Work out the finished part from the listing and answer in its coordinate system (mm). A direction names the side the tool comes from. Give positions to 0.01 mm unless a question says otherwise; leave off trailing zeros. Order: outer loops, then holes, each group sorted by start corner. A loop starts at its lowest first (then second) coordinate and runs counter-clockwise, first axis right, second up. Notation, with made-up numbers: (-32, 60.5) -> (-22, 60.5) arc R19 ccw to (-22, 81.5) -> close; hole circle Ø6 at (-31.5, 6.5). An arc over 180 degrees is marked (long way). Use a Markdown table: item, result. Add a question column.
```python
from build123d import *

# Parameters (mm, degrees)
BOSS_EXTRUDE1_DEPTH = 3.175
SKETCH3_R           = 3.3782
CUT_EXTRUDE2_DEPTH  = 4.175
SKETCH4_R           = 3.3782
CUT_EXTRUDE3_DEPTH  = 4.175
CHAMFER1_SIZE       = 3.175
CUT_EXTRUDE4_DEPTH  = 4.175


with BuildPart() as part:
    # Sketch1 → Boss-Extrude1 (new body)
    with BuildSketch(Plane(origin=(0, 0, 0), x_dir=(0, 0, -1), z_dir=(1, 0, 0))):
        with BuildLine():
            Line((118.405818623, 279.4), (147.442069819, 279.4))
            ThreePointArc((147.442069819, 279.4), (151.349937349, 278.055104531), (153.602474695, 274.590101219))
            Line((153.602474695, 274.590101219), (215.9, 25.4))
            Line((215.9, 25.4), (215.9, 0))
            Line((215.9, 0), (0, 0))
            Line((0, 0), (0, 25.4))
            Line((0, 25.4), (112.615117065, 275.655815701))
            ThreePointArc((112.615117065, 275.655815701), (114.95795187, 278.382421106), (118.405818623, 279.4))
        make_face()
    extrude(amount=BOSS_EXTRUDE1_DEPTH)

    # Sketch3 → Cut-Extrude2 (cut, through all)
    with BuildSketch(Plane(origin=(3.175, 0, 0), x_dir=(0, 0, -1), z_dir=(1, 0, 0))):
        with Locations((146.05, 244.475)):
            Circle(SKETCH3_R)
        with Locations((129.249479175, 225.425)):
            Circle(SKETCH3_R)
        with Locations((129.249479175, 263.525)):
            Circle(SKETCH3_R)
    extrude(amount=-CUT_EXTRUDE2_DEPTH, mode=Mode.SUBTRACT)

    # Sketch4 → Cut-Extrude3 (cut, through all)
    with BuildSketch(Plane(origin=(3.175, 0, 0), x_dir=(0, 0, -1), z_dir=(1, 0, 0))):
        with Locations((12.7, 12.7)):
            Circle(SKETCH4_R)
        with Locations((107.95, 12.7)):
            Circle(SKETCH4_R)
        with Locations((203.2, 12.7)):
            Circle(SKETCH4_R)
    extrude(amount=-CUT_EXTRUDE3_DEPTH, mode=Mode.SUBTRACT)

    # Chamfer1
    chamfer1_edges = [part.edges().sort_by_distance(p)[0] for p in [
        (1.5875, 0, -215.9),
        (1.5875, 0, 0),
    ]]
    chamfer(chamfer1_edges, length=CHAMFER1_SIZE)

    # Sketch5 → Cut-Extrude4 (cut, through all)
    with BuildSketch(Plane(origin=(3.175, 0, 0), x_dir=(0, 0, -1), z_dir=(1, 0, 0))):
        with BuildLine():
            Line((35.621183805, 25.4), (95.655352116, 25.4))
            ThreePointArc((95.655352116, 25.4), (103.688655638, 29.80722123), (104.287933788, 38.950438943))
            Line((104.287933788, 38.950438943), (73.736631302, 104.467918555))
            ThreePointArc((73.736631302, 104.467918555), (65.039859299, 109.967263315), (56.417997293, 104.351203163))
            Line((56.417997293, 104.351203163), (26.935131468, 38.833723552))
            ThreePointArc((26.935131468, 38.833723552), (27.622552146, 29.75319987), (35.621183805, 25.4))
        make_face()
        with BuildLine():
            Line((101.952143857, 205.538195526), (76.606881892, 149.21539116))
            ThreePointArc((76.606881892, 149.21539116), (74.370264914, 138.620954139), (76.749470333, 128.057624508))
            Line((76.749470333, 128.057624508), (102.005614522, 73.895648509))
            ThreePointArc((102.005614522, 73.895648509), (112.699783516, 68.621867985), (120.163196193, 77.921087453))
            Line((120.163196193, 77.921087453), (120.163196193, 201.629471974))
            ThreePointArc((120.163196193, 201.629471974), (112.637067937, 210.942373603), (101.952143857, 205.538195526))
        make_face()
        with BuildLine():
            Line((151.628803507, 203.939623803), (170.39715385, 128.866222433))
            ThreePointArc((170.39715385, 128.866222433), (171.039366508, 120.279332191), (168.775752137, 111.971313709))
            Line((168.775752137, 111.971313709), (151.020777865, 73.895648509))
            ThreePointArc((151.020777865, 73.895648509), (140.326608871, 68.621867985), (132.863196193, 77.921087453))
            Line((132.863196193, 77.921087453), (132.863196193, 201.629471974))
            ThreePointArc((132.863196193, 201.629471974), (141.224400607, 211.083106452), (151.628803507, 203.939623803))
        make_face()
        with BuildLine():
            Line((157.371040271, 25.4), (184.064314187, 25.4))
            ThreePointArc((184.064314187, 25.4), (191.571970984, 29.063198705), (193.304921501, 37.235151828))
            Line((193.304921501, 37.235151828), (183.988647407, 74.500248205))
            ThreePointArc((183.988647407, 74.500248205), (175.657972105, 81.671533437), (166.115458421, 76.21553532))
            Line((166.115458421, 76.21553532), (148.738458599, 38.950438943))
            ThreePointArc((148.738458599, 38.950438943), (149.337736749, 29.80722123), (157.371040271, 25.4))
        make_face()
    extrude(amount=-CUT_EXTRUDE4_DEPTH, mode=Mode.SUBTRACT)


solid = part.part
```
1) The part is cut by section D-D, the plane y = 178.5. Determine the outline of the cut face in (x, z) (3 decimals), then the cut area to 3 significant figures.
2) The part is cut by section A-A, the plane z = -203.2. Determine the outline of the cut face in (x, y) (3 decimals).
3) Straight lines are drawn through the part: line 1 (Z direction, x = 0.5, y = 64); line 2 (Z direction, x = 1.25, y = 92); line 3 (Z direction, x = 2.8, y = 154). For each, find the intervals that lie inside material, in ascending order.
4) Flat-ended cylindrical pins translate along their axes: pin 1 (8 mm diameter, centred on y = 162.5, z = -186.5, fed in from +X); pin 2 (1 mm diameter, centred on x = 2, y = 150.5, fed in from -Z); pin 3 (1.6 mm diameter, centred on x = 1.5, y = 121.5, fed in from +Z) (3 decimals); pin 4 (8 mm diameter, centred on y = 263.52, z = -129.25, fed in from -X). Find the tip coordinate at first contact, or state that the pin passes through.
5) Which of the six approach directions +Z, -Z, +X, -X, +Y, -Y give full straight-line access (tool end or side, diameter ignored) to faces 1 (the cylindrical face through (1.61, 81.654, -175.821)), 2 (the flat face through (1.57, 148.78, -55.52))?
6) Determine the mould class of faces 3 (the flat face through (1.61, 101.36, -89.2)), 4 (the flat face through (1.565, 151.739, -184.315)) for opening direction Y: released by +Y, released by -Y, zero draft, split by the parting line, or undercut.
7) The part is cut by section B-B, the plane y = 12.7. Determine the outline of the cut face in (x, z) (3 decimals).
8) The part is cut by section C-C, the plane z = -84. Determine the outline of the cut face in (x, y) (3 decimals), then the cut area to 3 significant figures.
A:
| question | item | result |
|---|---|---|
| 1 | outline | (0, -177.625) -> (3.175, -177.625) -> (3.175, -157.989) -> (0, -157.989) -> close; (0, -132.863) -> (3.175, -132.863) -> (3.175, -120.163) -> (0, -120.163) -> close; (0, -89.785) -> (3.175, -89.785) -> (3.175, -68.895) -> (0, -68.895) -> close |
| 1 | area | 169 mm^2 |
| 2 | outline | (0, 0) -> (3.175, 0) -> (3.175, 9.322) -> (0, 9.322) -> close; (0, 16.078) -> (3.175, 16.078) -> (3.175, 76.2) -> (0, 76.2) -> close |
| 3 | line 1 | -206.25 to -186.61, -160.42 to -92.61, -38.26 to -17.37 |
| 3 | line 2 | -199.25 to -159.46, -132.86 to -120.16, -93.56 to -79.55, -50.86 to -29.97 |
| 3 | line 3 | -183.75 to -164.11, -132.86 to -120.16, -78.76 to -57.87 |
| 4 | pin 1 | through |
| 4 | pin 2 | z = -184.75 |
| 4 | pin 3 | z = -42.885 |
| 4 | pin 4 | x = 0 |
| 5 | face 1 | +X, -X |
| 5 | face 2 | +Z, +X, -X, +Y |
| 6 | face 3 | undercut |
| 6 | face 4 | released by +Y |
| 7 | outline | (0, -215.9) -> (3.175, -215.9) -> (3.175, -206.578) -> (0, -206.578) -> close; (0, -199.822) -> (3.175, -199.822) -> (3.175, -111.328) -> (0, -111.328) -> close; (0, -104.572) -> (3.175, -104.572) -> (3.175, -16.078) -> (0, -16.078) -> close; (0, -9.322) -> (3.175, -9.322) -> (3.175, 0) -> (0, 0) -> close |
| 8 | outline | (0, 0) -> (3.175, 0) -> (3.175, 25.4) -> (0, 25.4) -> close; (0, 82.458) -> (3.175, 82.458) -> (3.175, 112.509) -> (0, 112.509) -> close; (0, 165.645) -> (3.175, 165.645) -> (3.175, 212.067) -> (0, 212.067) -> close |
| 8 | area | 323 mm^2 |
